Autodesk Inventor part; units mm, degrees
ref_plane "YZ Plane" through (0, 0, 0) normal (1, 0, 0) x (0, 1, 0)
ref_plane "XZ Plane" through (0, 0, 0) normal (0, 1, 0) x (-1, 0, 0)
ref_plane "XY Plane" through (0, 0, 0) normal (0, 0, 1) x (1, 0, 0)
sketch "Sketch1" plane through (0, 0, 0) normal (0, 0, 1) x (1, 0, 0)
  line L0 (-32.5, -26) -> (32.5, -26)
  line L1 (32.5, -26) -> (32.5, 26)
  line L2 (32.5, 26) -> (-32.5, 26)
  line L3 (-32.5, 26) -> (-32.5, -26)
  line L4 (-32.5, -26) -> (32.5, 26) construction
  line L5 (32.5, -26) -> (-32.5, 26) construction
  point P0 (0, 0)
  dimension "d0" = 65
  dimension "d1" = 52
extrude "Extrusion1" add sketch "Sketch1" along normal blind 1
sketch "Sketch4" plane through (0, 0, 1) normal (0, 0, 1) x (1, 0, 0)
  line L0 (29, -22.5) -> (16, -22.5) construction
  line L1 (16, -22.5) -> (16, 22.5) construction
  line L2 (16, 22.5) -> (29, 22.5) construction
  line L3 (29, 22.5) -> (29, -22.5) construction
  line L4 (29, -22.5) -> (16, 22.5) construction
  line L5 (16, -22.5) -> (29, 22.5) construction
  line L6 (32.5, -26) -> (32.5, 26)
  point P0 (0, 0)
  point P1 (22.5, 0)
  point P2 (22.5, 0)
  dimension "d20" = 13
  dimension "d31" = 3.5
  dimension "d32" = 45
hole "Hole3" at (16, 22.5, 1) at (29, 22.5, 1) at (16, -22.5, 1) direction (0, 0, -1) diameter 4.5 depth 8 tip angle 118
sketch "Sketch5" plane through (0, 0, 1) normal (0, 0, 1) x (1, 0, 0)
  circle A0 centre (16, 22.5) radius 2.25
  circle A1 centre (16, -22.5) radius 2.25
  point P0 (0, 0)
  point P1 (-25, -18.5)
  point P2 (0, 18.5)
  dimension "d33" = 4
  dimension "d34" = 4
  dimension "d35" = 41
  dimension "d36" = 16
hole "Hole4" at (-25, -18.5, 1) at (0, 18.5, 1) direction (0, 0, -1) diameter 4.5 depth 8 tip angle 118
sketch "Sketch6" plane through (0, 0, 1) normal (0, 0, 1) x (1, 0, 0)
  line L0 (32.5, -26) -> (32.5, 26)
  point P0 (0, 0)
  point P1 (22.5, 0)
  dimension "d44" = 10
hole "Hole5" at (22.5, 0, 1) direction (0, 0, -1) diameter 6.6 depth 8 tip angle 118
properties part number "CU5" material "Copper"
CAD build for the part. Positions are in the model's coordinates, mm. Round coordinates to 2 decimals unless told otherwise and drop trailing zeros. Write each loop counter-clockwise with the first axis right and the second up, starting at its lowest first coordinate (ties: lowest second). Pieces come first, ordered by that corner, then holes. Notation, with made-up numbers: (38, 28) -> (43, 28) arc R36 cw to (43, 66) -> close; hole circle Ø11 at (6, 49.25). An arc over 180 degrees is marked (long way). Answer in a Markdown table with one row per item. Add a question column.
Item 1: Saw through at C-C, the plane z = 0.45. Write the cut outline in (x, y).
Item 2: Mould opens along X. For faces 1 (the face through (16.86, 20.42, 0.49)), 2 (the face through (0, 0, 0)) say: pulls with the +X half, pulls with the -X half, needs draft (parallel to the pull), parting line crosses it, or undercut.
Item 3: Drill centre lines: line 1 (Y direction, x = 16, z = 0.1); line 2 (X direction, y = 22.5, z = 0.3); line 3 (Y direction, x = 14, z = 0.95). Where is each one in solid material? Low to high. Write a range as from..to.
Item 4: Saw through at A-A, the plane x = -25. Write the cut outline in (y, z), then the cut area to 3 significant figures.
Item 5: Saw through at D-D, the plane y = 0. Write the cut outline in (x, z), then the cut area to 3 significant figures.
Item 6: Saw through at B-B, the plane x = 16. Write the cut outline in (y, z), then the cut area to 3 significant figures.
Findings below:
| question | item | result |
|---|---|---|
| 1 | outline | (-32.5, -26) -> (32.5, -26) -> (32.5, 26) -> (-32.5, 26) -> close; hole circle Ø4.5 at (-25, -18.5); hole circle Ø4.5 at (0, 18.5); hole circle Ø4.5 at (16, -22.5); hole circle Ø4.5 at (16, 22.5); hole circle Ø6.6 at (22.5, 0); hole circle Ø4.5 at (29, 22.5) |
| 2 | face 1 | undercut |
| 2 | face 2 | needs draft |
| 3 | line 1 | y = -26..-24.75, -20.25..20.25, 24.75..26 |
| 3 | line 2 | x = -32.5..13.75, 18.25..26.75, 31.25..32.5 |
| 3 | line 3 | y = -26..-23.53, -21.47..21.47, 23.53..26 |
| 4 | outline | (-26, 0) -> (-20.75, 0) -> (-20.75, 1) -> (-26, 1) -> close; (-16.25, 0) -> (26, 0) -> (26, 1) -> (-16.25, 1) -> close |
| 4 | area | 47.5 mm^2 |
| 5 | outline | (-32.5, 0) -> (19.2, 0) -> (19.2, 1) -> (-32.5, 1) -> close; (25.8, 0) -> (32.5, 0) -> (32.5, 1) -> (25.8, 1) -> close |
| 5 | area | 58.4 mm^2 |
| 6 | outline | (-26, 0) -> (-24.75, 0) -> (-24.75, 1) -> (-26, 1) -> close; (-20.25, 0) -> (20.25, 0) -> (20.25, 1) -> (-20.25, 1) -> close; (24.75, 0) -> (26, 0) -> (26, 1) -> (24.75, 1) -> close |
| 6 | area | 43.0 mm^2 |
